Design review of the part built by this model. Coordinates are the model's own, in mm. A direction names the side the tool comes from. Coordinates: 2 decimals unless noted, no trailing zeros. Write each loop counter-clockwise with the first axis right and the second up, starting at its lowest first coordinate (ties: lowest second). Pieces come first, ordered by that corner, then holes. Notation, with made-up numbers: (50.5, -22.5) -> (73.5, -22.5) arc R18 cw to (73.5, -12.5) -> close; hole circle Ø6 at (-39, 7.25). An arc over 180 degrees is marked (long way). Answer in a Markdown table with one row per item. Add a question column.
Item 1: Take a section at C-C, the plane y = 61.5. Write out the cut boundary in (x, z), and give its area (3 significant figures).
Item 2: Take a section at B-B, the plane z = 15. Write out the cut boundary in (x, y), and give its area (3 significant figures).
Item 3: For faces 1 (the face through (10, 19.05, 44)), 2 (the face through (12, -19, 50.8)), 3 (the face through (10, 84, 0)), list the 3-axis set-ups (+Z, -Z, +X, -X, +Y, -Y) from which the entire face can be reached by the end or side of a thin tool; tool diameter is ignored.
Item 4: Take a section at A-A, the plane x = 14. Write out the cut boundary in (y, z), and give its area (3 significant figures).
Item 5: Clearance check with flat-ended pins moving along their axes: P1, Ø8, axis at x = -1, y = 73.5, coming from the +Z side; P2, Ø8, axis at x = 4.5, y = 40.5, coming from the -Z side; P3, Ø10, axis at y = 86.5, z = 10.5, coming from the -X side; P4, Ø5.5, axis at x = 7.5, z = 17, coming from the -Y side. State where each tip first meets the part, or that it passes through.
Item 6: Draft analysis for pull direction Y (two halves, no side actions). For faces 4 (the face through (9, -38.1, 60)), 5 (the face through (19.05, 56, 17)), 6 (the face through (-2, 129, 9)), state which applies: released by +Y, released by -Y, zero draft, split by the parting line, or undercut.
Item 7: To check wall thickness, follow line 1 (Y direction, x = 9.25, z = 66.5); line 2 (X direction, y = -19.05, z = 62.5) (3 decimals); line 3 (Y direction, x = 10.25, z = 40). State the ranges of each line that lie inside material, in increasing order.
Autodesk Fusion 360 part; units mm, degrees
sketch "Sketch1" plane through (0, 0, 0) normal (0, 0, 1) x (1, 0, 0)
  line L0 (0, 0) -> (19.05, 0)
  line L1 (19.05, 0) -> (19.05, 165.1)
  line L2 (19.05, 165.1) -> (0, 165.1)
  line L3 (0, 165.1) -> (0, 0)
  line L4 (0, 165.1) -> (-5, 162.5)
  line L5 (-5, 162.5) -> (0, 160)
  line L6 (-5, 157.5) -> (0, 160)
  line L7 (-5, 157.5) -> (0, 155)
  line L8 (0, 155) -> (-5, 152.5)
  line L9 (-5, 152.5) -> (0, 150)
  line L10 (0, 150) -> (-5, 147.5)
  line L11 (-5, 147.5) -> (0, 145)
  line L12 (0, 145) -> (-5, 142.5)
  line L13 (-5, 142.5) -> (0, 140)
  line L14 (0, 140) -> (-5, 137.5)
  line L15 (-5, 137.5) -> (0, 135)
  line L16 (0, 135) -> (-5, 132.5)
  line L17 (-5, 132.5) -> (0, 130)
  line L18 (0, 130) -> (-5, 127.5)
  line L19 (-5, 127.5) -> (0, 125)
  line L20 (0, 125) -> (-5, 122.5)
  line L21 (-5, 122.5) -> (0, 120)
  dimension "d2" = 19.05
  dimension "d3" = 165.1
extrude "Extrude1" add sketch "Sketch1" along normal blind 19.05 contours L0 L1 L2 L3 | L3 L20 L21 | L3 L18 L19 | L3 L16 L17 | L3 L14 L15 | L3 L8 L9 | L3 L12 L13 | L3 L10 L11
sketch "Sketch2" plane through (0, 0, 19.05) normal (0, 0, 1) x (-1, 0, 0)
  line L0 (5, -122.5) -> (0, -120)
  line L1 (0, -120) -> (0, 0)
  line L2 (0, 0) -> (-19.05, 0)
  line L3 (-19.05, 0) -> (-19.05, -165.1)
  line L4 (-19.05, -165.1) -> (0, -165.1)
  line L5 (0, -165.1) -> (0, -155)
  line L6 (0, -155) -> (5, -152.5)
  line L7 (5, -152.5) -> (0, -150)
  line L8 (0, -150) -> (5, -147.5)
  line L9 (5, -147.5) -> (0, -145)
  line L10 (0, -145) -> (5, -142.5)
  line L11 (5, -142.5) -> (0, -140)
  line L12 (0, -140) -> (5, -137.5)
  line L13 (5, -137.5) -> (0, -135)
  line L14 (0, -135) -> (5, -132.5)
  line L15 (5, -132.5) -> (0, -130)
  line L16 (0, -130) -> (5, -127.5)
  line L17 (5, -127.5) -> (0, -125)
  line L18 (0, -125) -> (5, -122.5)
  line L19 (0, 0) -> (-19.05, 0)
  line L20 (-19.05, 0) -> (-19.05, -19.05)
  line L21 (-19.05, -19.05) -> (0, -19.05)
  line L22 (0, -19.05) -> (0, 0)
  dimension "d6" = 19.05
  dimension "d7" = 19.05
extrude "Extrude2" add sketch "Sketch2" along normal blind 50.8 contours L1 L2 L3 L19 L20 L21 L22
sketch "Sketch3" plane through (0, 0, 0) normal (0, -1, 0) x (1, 0, 0)
  line L0 (0, 0) -> (19.05, 0)
  line L1 (19.05, 0) -> (19.05, 69.85)
  line L2 (19.05, 69.85) -> (0, 69.85)
  line L3 (0, 69.85) -> (0, 0)
  line L4 (0, 69.85) -> (19.05, 69.85)
  line L5 (19.05, 69.85) -> (19.05, 50.8)
  line L6 (19.05, 50.8) -> (0, 50.8)
  line L7 (0, 50.8) -> (0, 69.85)
  dimension "d10" = 19.05
extrude "Extrude3" add sketch "Sketch3" along normal blind 38.1 contours L1 L2 L3 L4 L5 L6 L7
extrude "Extrude4" add sketch "Sketch1" along normal blind 19.05 contours L3 L4 L5 | L3 L6 L7
sketch "Sketch4" plane through (0, 0, 69.85) normal (0, 0, 1) x (-1, 0, 0)
  line L0 (0, -19.05) -> (0, 38.1)
  line L1 (0, 38.1) -> (-19.05, 38.1)
  line L2 (-19.05, 38.1) -> (-19.05, -19.05)
  line L3 (-19.05, -19.05) -> (0, -19.05)
  circle A0 centre (-9.525, 19.05) radius 1
  circle A1 centre (-9.525, 31.75) radius 1.0988
  dimension "d15" = 12.7
  dimension "d16" = 9.525
  dimension "d17" = 6.35
extrude "Extrude5" cut sketch "Sketch4" against normal blind 33 contours A0 | A1
Answers:
| question | item | result |
|---|---|---|
| 1 | outline | (0, 0) -> (19.05, 0) -> (19.05, 19.05) -> (0, 19.05) -> close |
| 1 | area | 363 mm^2 |
| 2 | outline | (-5, 122.5) -> (0, 120) -> (0, 0) -> (19.05, 0) -> (19.05, 165.1) -> (0, 165.1) -> (-5, 162.5) -> (0, 160) -> (-5, 157.5) -> (0, 155) -> (-5, 152.5) -> (0, 150) -> (-5, 147.5) -> (0, 145) -> (-5, 142.5) -> (0, 140) -> (-5, 137.5) -> (0, 135) -> (-5, 132.5) -> (0, 130) -> (-5, 127.5) -> (0, 125) -> close |
| 2 | area | 3,260 mm^2 |
| 3 | face 1 | +Z, +X, -X, +Y |
| 3 | face 2 | -Z, +X, -X, -Y |
| 3 | face 3 | -Z, +X, -X, +Y, -Y |
| 4 | outline | (-38.1, 50.8) -> (0, 50.8) -> (0, 0) -> (165.1, 0) -> (165.1, 19.05) -> (19.05, 19.05) -> (19.05, 69.85) -> (-38.1, 69.85) -> close |
| 4 | area | 4,840 mm^2 |
| 5 | P1 | stops at z = 19.05 |
| 5 | P2 | stops at z = 0 |
| 5 | P3 | stops at x = 0 |
| 5 | P4 | stops at y = 0 |
| 6 | face 4 | released by -Y |
| 6 | face 5 | zero draft |
| 6 | face 6 | undercut |
| 7 | line 1 | y = -38.1 to -32.81, -30.69 to -20.01, -18.09 to 19.05 |
| 7 | line 2 | x = 0 to 8.525, 10.525 to 19.05 |
| 7 | line 3 | y = 0 to 19.05 |
